Source: CAD feature listing. Evaluate the final solid. Frame: model axes, mm. A direction names the side the tool comes from. Round coordinates to 2 decimals unless told otherwise and drop trailing zeros. Loops run counter-clockwise (first coordinate to the right, second up) from the corner with the lowest first, then second, coordinate; pieces in that order, holes last. Notation, with made-up numbers: (-10.5, -7.75) -> (36.5, -7.75) arc R26 ccw to (36.5, 6.25) -> close; hole circle Ø7 at (27, 76). An arc over 180 degrees is marked (long way). Put each result on its own line as item: value. Start each with the question number.
1. Material intervals for L1, parallel to X at y = -23.75, z = -17; L2, parallel to Y at x = 1, z = -5.5; L3, parallel to X at y = -24.75, z = -6, sorted ascending.
2. Cut plane B-B (x = 4.5). Return the cut outline in (y, z).
3. Draft query along Y for faces 3 (the flat face through (0, -11.485, -7)), 4 (the cylindrical face through (6.074, -11.72, -7.228)), 5 (the flat face through (-7.5, -20, -7)). Return one class per face: pulls with the +Y half, pulls with the -Y half, needs draft (parallel to the pull), parting line crosses it, or undercut.
4. Cut plane D-D (z = 4). Return the cut outline in (x, y), then the cut area to 3 significant figures.
5. Contact query for flat-ended pins moving along their axis: pin 1 (4 mm diameter, centred on x = -5.5, z = -13.5, fed in from -Y); pin 2 (4 mm diameter, centred on x = 3, y = -13.5, fed in from -Z); pin 3 (1 mm diameter, centred on x = -4, z = 2.5, fed in from +Y); pin 4 (2.5 mm diameter, centred on x = -3.5, y = -23.75, fed in from +Z). Output: stop coordinate, or through.
6. Cut plane A-A (y = -12). Return the cut outline in (x, z).
7. Set-up query: faces 1 (the flat face through (1.77, -12.52, 4.27)), 2 (the flat face through (-1.5, -12, -7)). Return all of +Z, -Z, +X, -X, +Y, -Y with unobstructed straight access to the full face (end or side cutting, diameter ignored); none if empty.
8. Cut plane C-C (z = -10). Return the cut outline in (x, y), then the cut area to 3 significant figures.
```python
from build123d import *

# Parameters (mm, degrees)
BOSS_EXTRUDE2_DEPTH = 7.5
FILLET2_R           = 5
SKETCH4_R           = 2
SKETCH4_W           = 3
SKETCH4_H           = 2
CUT_EXTRUDE1_DEPTH  = 100
FILLET3_R           = 5
FILLET4_R           = 5


with BuildPart() as part:
    # Sketch2 → Boss-Extrude2 (new, symmetric)
    with BuildSketch(Plane(origin=(0, 0, 0), x_dir=(0, 0, -1), z_dir=(1, 0, 0))):
        Polygon((-7.967160281, -29.21673477), (-7.967160281, -16.21673477), (-1.967160281, -10.21673477), (16.032839719, -10.21673477), (22.032839719, -16.21673477), (22.032839719, -29.21673477), align=None)
    extrude(amount=BOSS_EXTRUDE2_DEPTH, both=True)

    # Fillet2
    fillet2_edges = [part.edges().sort_by_distance(p)[0] for p in [
        (0, -16.21673477, 7.967160281),
        (0, -16.21673477, -22.032839719),
    ]]
    fillet(fillet2_edges, radius=FILLET2_R)

    # Sketch4 → Cut-Extrude1 (cut, symmetric)
    with BuildSketch(Plane.XY):
        with Locations(Location((-3.5, -23.752268676, 0), (0, 0, 90))):
            Circle(SKETCH4_R)
        with Locations(Location((3.5, -23.752268676, 0), (0, 0, 90))):
            Circle(SKETCH4_R)
        with Locations((0, -12.484501723)):
            Rectangle(SKETCH4_W, SKETCH4_H)
    extrude(amount=CUT_EXTRUDE1_DEPTH, both=True, mode=Mode.SUBTRACT)

    # Fillet3
    fillet3_edges = [part.edges().sort_by_distance(p)[0] for p in [
        (7.5, -29.21673477, -7.032839719),
        (-7.5, -29.21673477, -7.032839719),
    ]]
    fillet(fillet3_edges, radius=FILLET3_R)

    # Fillet4
    fillet4_edges = [part.edges().sort_by_distance(p)[0] for p in [
        (7.5, -10.21673477, -7.032839719),
        (-7.5, -10.21673477, -7.032839719),
    ]]
    fillet(fillet4_edges, radius=FILLET4_R)


solid = part.part
```
Solution:
1. L1: x = -7.5 to -5.5, -1.5 to 1.5, 5.5 to 7.5
1. L2: y = -29.22 to -13.48, -11.48 to -10.22
1. L3: x = -7.47 to -5.23, -1.77 to 1.77, 5.23 to 7.47
2. outline: (-28.8, -22.03) -> (-25.48, -22.03) -> (-25.48, 7.97) -> (-28.8, 7.97) -> close; (-22.02, -22.03) -> (-18.29, -22.03) arc R5 ccw to (-14.75, -20.57) -> (-10.63, -16.45) -> (-10.63, 2.38) -> (-14.75, 6.5) arc R5 ccw to (-18.29, 7.97) -> (-22.02, 7.97) -> close
3. face 3: undercut
3. face 4: pulls with the +Y half
3. face 5: needs draft
4. outline: (-7.5, -24.22) arc R5 ccw to (-2.5, -29.22) -> (2.5, -29.22) arc R5 ccw to (7.5, -24.22) -> (7.5, -15.22) arc R5 ccw to (6.52, -12.25) -> (1.5, -12.25) -> (1.5, -13.48) -> (-1.5, -13.48) -> (-1.5, -12.25) -> (-6.52, -12.25) arc R5 ccw to (-7.5, -15.22) -> close; hole circle Ø4 at (-3.5, -23.75); hole circle Ø4 at (3.5, -23.75)
4. area: 213 mm^2
5. pin 1: stops at y = -29.12
5. pin 2: stops at z = -21.18
5. pin 3: stops at y = -10.36
5. pin 4: passes through
6. outline: (-6.33, -17.82) -> (-1.5, -17.82) -> (-1.5, 3.75) -> (-6.33, 3.75) -> close; (1.5, -17.82) -> (6.33, -17.82) -> (6.33, 3.75) -> (1.5, 3.75) -> close
7. face 1: +Z, +X, -X, +Y
7. face 2: +Z, -Z
8. outline: (-7.5, -24.22) arc R5 ccw to (-2.5, -29.22) -> (2.5, -29.22) arc R5 ccw to (7.5, -24.22) -> (7.5, -15.22) arc R5 ccw to (2.5, -10.22) -> (-2.5, -10.22) arc R5 ccw to (-7.5, -15.22) -> close; hole circle Ø4 at (-3.5, -23.75); hole (-1.5, -13.48) -> (1.5, -13.48) -> (1.5, -11.48) -> (-1.5, -11.48) -> close; hole circle Ø4 at (3.5, -23.75)
8. area: 232 mm^2
